The figure shows three views and two pictorial views of one solid part (mm, origin at its lowest corner). Answer the questions. A direction names the side the tool comes from. Round coordinates to 2 decimals unless told otherwise and drop trailing zeros. Write each loop counter-clockwise with the first axis right and the second up, starting at its lowest first coordinate (ties: lowest second). Pieces come first, ordered by that corner, then holes. Notation, with made-up numbers: M 59,34.25 L 67,34.25 A37 ccw 67,73.25 Z; hole C -30,-32.75 d4. An arc over 180 degrees is marked long. Answer in a Markdown table with one row per item.
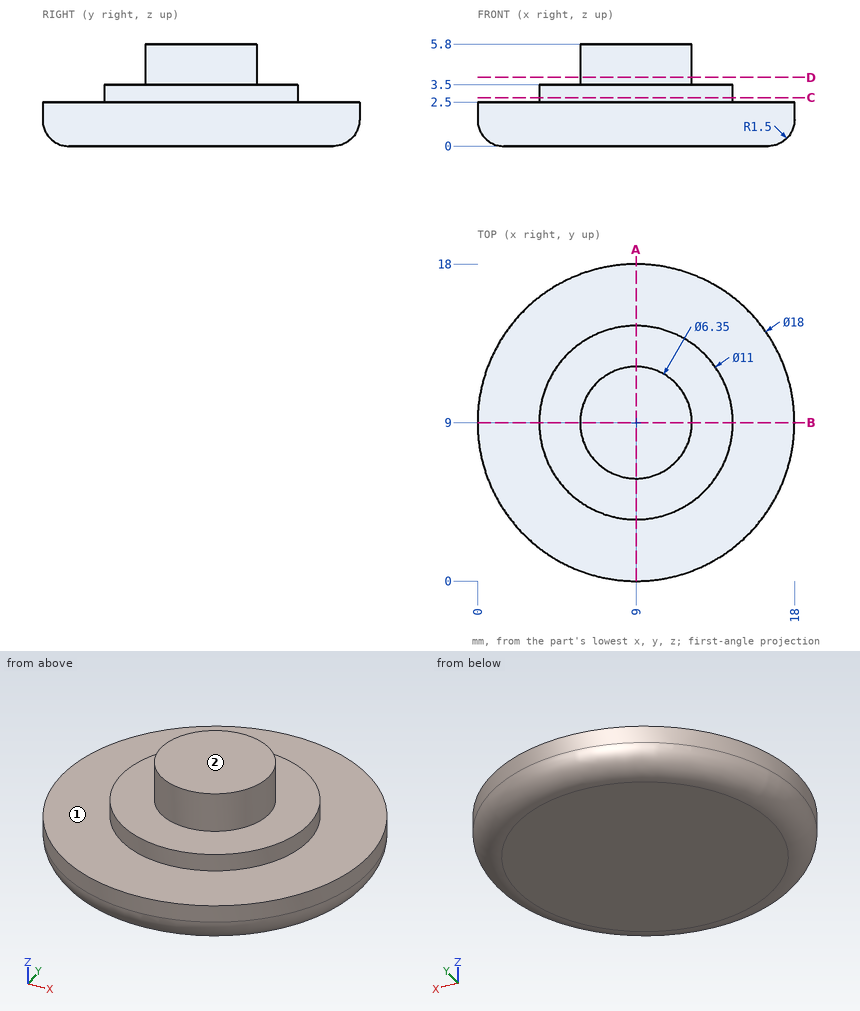
1. A tool of negligible diameter and unlimited length cuts with its end or side. For the marked faces 1 and 2, from which of +Z, -Z, +X, -X, +Y, -Y can it reach the whole face along a straight path? Write none if from no direction.
Calculated:
| item | result |
|---|---|
| face 1 | +Z |
| face 2 | +Z, +X, -X, +Y, -Y |
2. Given pin 1 (1 mm diameter, centred on y = 5.5, z = 1.5, fed in from -X); pin 2 (3 mm diameter, centred on x = 14, y = 15.5, fed in from +Z); pin 3 (2 mm diameter, centred on x = 6, y = 13.5, fed in from +Z), each flat-ended and moving along its own axis, determine where each tip first touches the part or whether it passes through.
Calculated:
| item | result |
|---|---|
| pin 1 | stops at x = 0.51 |
| pin 2 | stops at z = 2.5 |
| pin 3 | stops at z = 3.5 |
3. The part is cut by section D-D (z = 3.9). Determine the outline of the cut face in (x, y) (3 decimals), plus the area to 3 significant figures.
Calculated:
| item | result |
|---|---|
| outline | C 9,9 d6.35 |
| area | 31.7 mm² |
4. Consider line 1 along Z through (x, y) = (13.75, 13); line 2 along Y through (x, z) = (9, 4) (3 decimals); line 3 along X through (y, z) = (13.5, 1.6). Determine where each line is inside the solid, lowest interval first. Write a range as from..to.
Calculated:
| item | result |
|---|---|
| line 1 | z = 0..2.5 |
| line 2 | y = 5.825..12.175 |
| line 3 | x = 1.21..16.79 |
5. The part is cut by section A-A (x = 9). Determine the outline of the cut face in (y, z) (3 decimals), plus the area to 3 significant figures.
Calculated:
| item | result |
|---|---|
| outline | M 0,1.5 A1.5 ccw 1.5,0 L 16.5,0 A1.5 ccw 18,1.5 L 18,2.5 L 14.5,2.5 L 14.5,3.5 L 12.175,3.5 L 12.175,5.8 L 5.825,5.8 L 5.825,3.5 L 3.5,3.5 L 3.5,2.5 L 0,2.5 Z |
| area | 69.6 mm² |
6. The part is cut by section C-C (z = 2.75). Determine the outline of the cut face in (x, y), plus the area to 3 significant figures.
Calculated:
| item | result |
|---|---|
| outline | C 9,9 d11 |
| area | 95.0 mm² |
